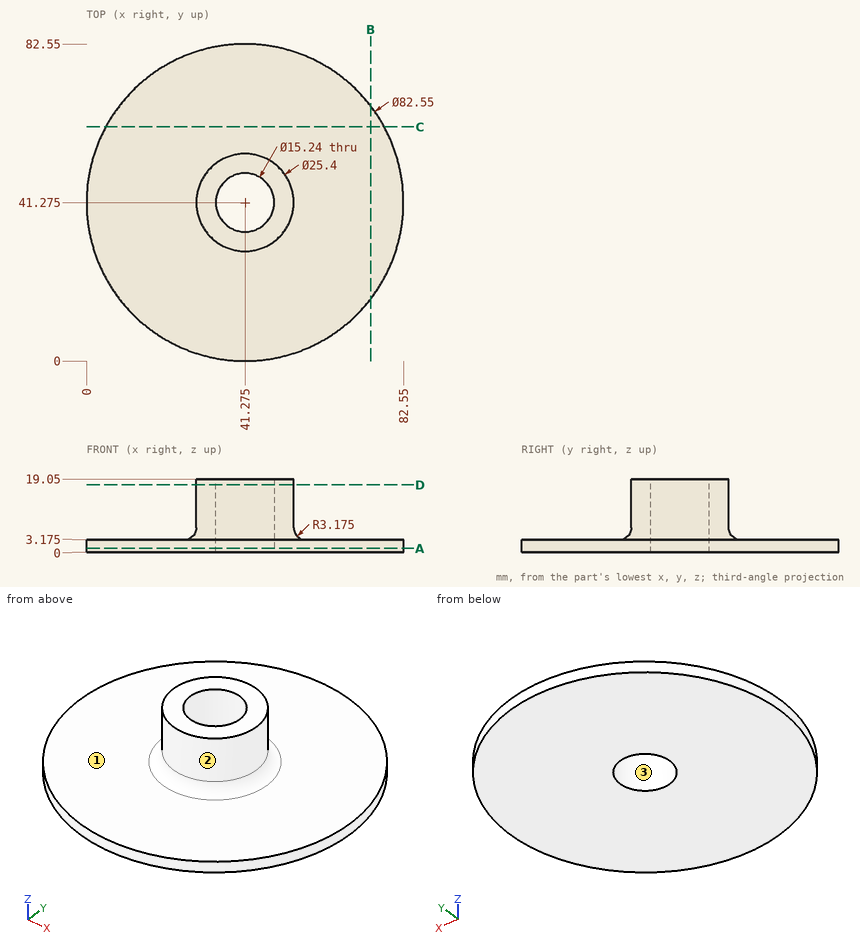
Source: three-view drawing plus pictorial views. Frame: mm from the lowest corner of the part. Coordinates: 2 decimals unless noted, no trailing zeros. Order: outer loops, then holes, each group sorted by start corner. A loop starts at its lowest first (then second) coordinate and runs counter-clockwise, first axis right, second up. Notation, with made-up numbers: M 29,-15.75 L 83,-15.75 A22 ccw 83,-5.75 Z; hole C 62.25,16 d7. An arc over 180 degrees is marked long. One line per question, with ' | ' between items. Start each with the question number.
Item 1: Cut plane C-C, the plane y = 61. Return the cut outline in (x, z) (3 decimals), then the cut area to 3 significant figures.
Item 2: Cut plane A-A, the plane z = 1. Return the cut outline in (x, y) (3 decimals).
Item 3: Draft query along Y for the marked faces 1, 2 and 3. Return one class per face: released by +Y, released by -Y, zero draft, split by the parting line, or undercut.
Item 4: Pin query (flat end, axial travel): pin 1 Ø6 at (x, z) = (18, 4) entering from +Y; pin 2 Ø12 at (x, y) = (41.275, 41.275) entering from +Z; pin 3 Ø6 at (x, z) = (20.5, 6) entering from -Y; pin 4 Ø3 at (x, y) = (25, 32) entering from +Z (3 decimals). Return the tip coordinate at first contact, or that it passes through.
Item 5: Ray query, probe 1 along Y at (x, z) = (41.5, 8); probe 2 along Z at (x, y) = (70.5, 59) (3 decimals); probe 3 along Y at (x, z) = (35.5, 7.75). Return the intervals inside material, ascending. Write a range as [from, to].
Item 6: Cut plane D-D, the plane z = 17.5. Return the cut outline in (x, y) (3 decimals).
Item 7: Cut plane B-B, the plane x = 74. Return the cut outline in (y, z) (3 decimals).
A:
1) outline: M 5.018,0 L 77.532,0 L 77.532,3.175 L 5.018,3.175 Z | area: 230 mm2
2) outline: C 41.275,41.275 d82.55; hole C 41.275,41.275 d15.24
3) face 1: zero draft | face 2: split by the parting line | face 3: undercut
4) pin 1: stops at y = 77.16 | pin 2: passes through | pin 3: stops at y = 5.04 | pin 4: stops at z = 3.175
5) probe 1: y = [28.58, 33.66], [48.89, 53.97] | probe 2: z = [0, 3.175] | probe 3: y = [29.96, 36.3], [46.25, 52.59]
6) outline: C 41.275,41.275 d25.4; hole C 41.275,41.275 d15.24
7) outline: M 16.121,0 L 66.429,0 L 66.429,3.175 L 16.121,3.175 Z
